Check sheet for the drawn part. Datum: minimum x, y, z corner. Units: mm. Give positions to 0.01 mm unless a question says otherwise; leave off trailing zeros. Order: outer loops, then holes, each group sorted by start corner. A loop starts at its lowest first (then second) coordinate and runs counter-clockwise, first axis right, second up.
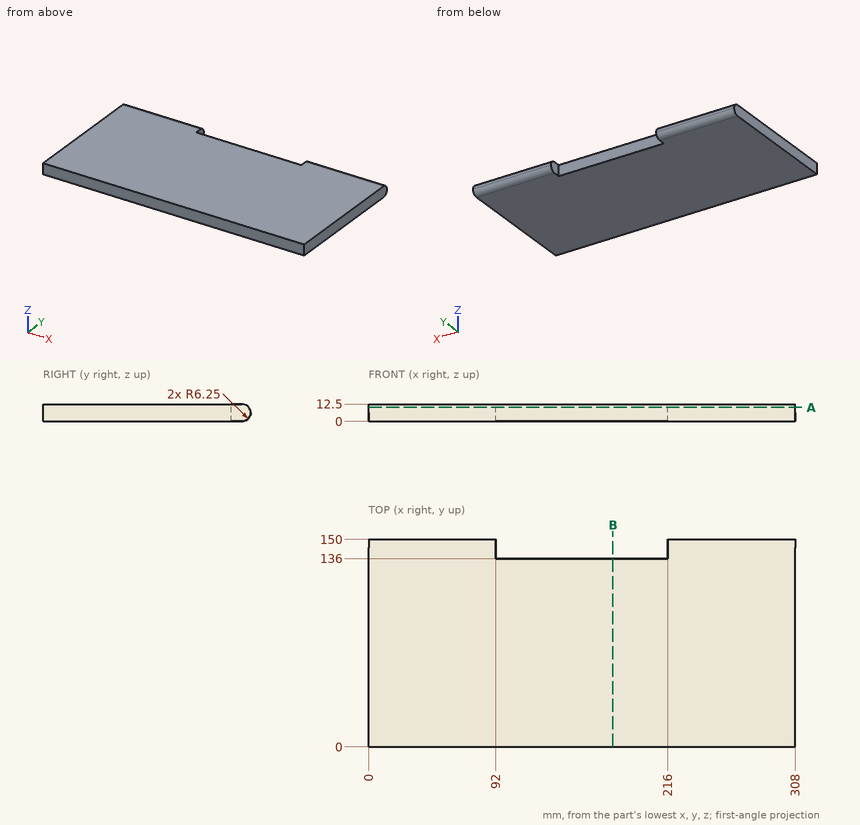
Item 1: Sectioned sample at A-A (z = 10). Enter the section's corners in (x, y).
Reported:
outline: (0, 0) - (308, 0) - (308, 148.75) - (216, 148.75) - (216, 136) - (92, 136) - (92, 148.75) - (0, 148.75) - close
Item 2: Gauge pin test, flat ends, axial feed: pin 1 (6 mm diameter, centred on x = 110, z = 8, fed in from +Y); pin 2 (5 mm diameter, centred on x = 232.5, z = 10, fed in from +Y). Record the tip position at first contact, or that the pin passes through.
Reported:
pin 1: stops at y = 136
pin 2: stops at y = 149.87
Item 3: Sectioned sample at B-B (x = 176.5). Enter the section's corners in (y, z).
Reported:
outline: (0, 0) - (136, 0) - (136, 12.5) - (0, 12.5) - close
Item 4: Scan lines: L1, parallel to X at y = 141, z = 4.5; L2, parallel to Y at x = 116.5, z = 12; L3, parallel to Y at x = 88.5, z = 6.5 (3 decimals). Record each from-to range of solid material in increasing order.
Reported:
L1: x = 0 to 92, 216 to 308
L2: y = 0 to 136
L3: y = 0 to 149.995
